Geometry: final body of the model. Coordinates: model frame, mm. A direction names the side the tool comes from. Round coordinates to 2 decimals unless told otherwise and drop trailing zeros. Write each loop counter-clockwise with the first axis right and the second up, starting at its lowest first coordinate (ties: lowest second). Pieces come first, ordered by that corner, then holes. Notation, with made-up numbers: M 23,61 L 58,61 A17 ccw 58,86 Z; hole C 62,9 d1. An arc over 180 degrees is marked long. Answer as CSV lines item,"result". Start each with the question number.
Q1. First-contact query: pin 1 (12 mm diameter, centred on x = -3.5, z = 145.5, fed in from -Y); pin 2 (6 mm diameter, centred on x = -8, z = 30.5, fed in from +Y) (3 decimals); pin 3 (1.6 mm diameter, centred on x = -1.5, y = 13.5, fed in from -Z); pin 4 (2.5 mm diameter, centred on x = -1.5, z = 53.5, fed in from +Y) (3 decimals). Flat tips, straight axial feed; report the tip coordinate or a pass-through.
Q2. Ray query, probe 1 along Y at (x, z) = (-24, 13) (3 decimals); probe 2 along X at (y, z) = (22, 149.5) (3 decimals); probe 3 along X at (y, z) = (2.1, 85). Return the intervals inside material, ascending.
Q3. Mould query, pull axis Z, two halves, no side actions, for faces 4 (the flat face through (-1.61, 23.376, 158.009)), 5 (the flat face through (-2, 14, 145)), 6 (the cylindrical face through (-13.837, 1.565, 157.615)), 7 (the flat face through (-20, 0, 84)). Classes: pulls with the +Z half, pulls with the -Z half, needs draft (parallel to the pull), parting line crosses it, or undercut.
Q4. Section query C-C on x = -9.75. Output: boundary loops of the cut face in (y, z) (3 decimals).
Q5. Reachability of faces 1 (the flat face through (-17.3, 3.175, 83.8)), 2 (the cylindrical face through (-1.565, 13.578, 154.835)), 3 (the flat face through (-2, 9, 10)) from +Z, -Z, +X, -X, +Y, -Y: full face, straight path, thin tool, end or side. Return the list, or none.
Q6. Section query D-D on z = 148. Output: boundary loops of the cut face in (x, y) (3 decimals), and give its area (3 significant figures).
Q7. Section query B-B on z = 109.5. Output: boundary loops of the cut face in (x, y) (3 decimals), and give its area (3 significant figures).
```python
from build123d import *

# Parameters (mm, degrees)
BASE_FLANGE1_DEPTH = 170
FILLET1_R          = 5
SKETCH6_R          = 2
CUT_EXTRUDE1_DEPTH = 178.200451467
SKETCH7_R          = 2.5
CUT_EXTRUDE2_DEPTH = 178.200451467
CUT_EXTRUDE3_DEPTH = 177.690635363
FILLET2_R          = 5
CUT_EXTRUDE4_DEPTH = 175.263907966
FILLET3_R          = 7


# Sheet-metal steps are written as plain solids
with BuildPart() as part:
    # Sketch1 → Base-Flange1 (new body)
    with BuildSketch(Plane.XY):
        with BuildLine():
            Line((0, 40), (0, 4.175))
            ThreePointArc((0, 4.175), (-1.222829189, 1.222829189), (-4.175, 0))
            Line((-4.175, 0), (-30, 0))
            Line((-30, 0), (-30, 3.175))
            Line((-30, 3.175), (-4.175, 3.175))
            ThreePointArc((-4.175, 3.175), (-3.467893219, 3.467893219), (-3.175, 4.175))
            Line((-3.175, 4.175), (-3.175, 40))
            Line((-3.175, 40), (0, 40))
        make_face()
    extrude(amount=BASE_FLANGE1_DEPTH)

    # Fillet1
    fillet1_edges = [part.edges().sort_by_distance(p)[0] for p in [
        (-1.5875, 40, 170),
        (-1.5875, 40, 0),
        (-30, 1.5875, 170),
        (-30, 1.5875, 0),
    ]]
    fillet(fillet1_edges, radius=FILLET1_R)

    # Sketch6 → Cut-Extrude1 (cut, through all)
    with BuildSketch(Plane.ZY):
        with BuildLine():
            ThreePointArc((159.640076561, 18.14476706), (156.999504521, 20.49580498), (154.648466601, 17.85523294))
            ThreePointArc((154.648466601, 17.85523294), (154.837103455, 13.516938304), (154.9, 9.175))
            ThreePointArc((154.9, 9.175), (157.4, 6.675), (159.9, 9.175))
            ThreePointArc((159.9, 9.175), (159.835005505, 13.661766133), (159.640076561, 18.14476706))
        make_face()
        with Locations(Location((5, 9.175, 0), (0, 0, 180))):
            Circle(SKETCH6_R)
    extrude(amount=CUT_EXTRUDE1_DEPTH, mode=Mode.SUBTRACT)

    # Sketch7 → Cut-Extrude2 (cut, through all)
    with BuildSketch(Plane.XZ):
        with Locations(Location((-14.5875, 160, 0), (0, 0, 270))):
            Circle(SKETCH7_R)
        with Locations(Location((-14.5875, 85, 0), (0, 0, 270))):
            Circle(SKETCH7_R)
        with Locations(Location((-14.5875, 10, 0), (0, 0, 270))):
            Circle(SKETCH7_R)
    extrude(amount=-CUT_EXTRUDE2_DEPTH, mode=Mode.SUBTRACT)

    # Sketch8 → Cut-Extrude3 (cut, through all)
    with BuildSketch(Plane.ZY.offset(3.175)):
        with BuildLine():
            Line((0, 12.85080004), (170, 24.175))
            Line((170, 24.175), (170, 35))
            ThreePointArc((170, 35), (168.535533906, 38.535533906), (165, 40))
            Line((165, 40), (5, 40))
            ThreePointArc((5, 40), (1.464466094, 38.535533906), (0, 35))
            Line((0, 35), (0, 12.85080004))
        make_face()
    extrude(amount=-CUT_EXTRUDE3_DEPTH, mode=Mode.SUBTRACT)

    # Fillet2
    fillet2_edges = [part.edges().sort_by_distance(p)[0] for p in [
        (-1.5875, 24.175, 170),
        (-1.5875, 12.85080004, 0),
    ]]
    fillet(fillet2_edges, radius=FILLET2_R)

    # Sketch9 → Cut-Extrude4 (cut, through all)
    with BuildSketch(Plane(origin=(0, 0, 0), x_dir=(0, 0, -1), z_dir=(1, 0, 0))):
        Polygon((-10, 13.51692945), (-145, 22.509676476), (-145, 4.175), (-10, 4.175), align=None)
    extrude(amount=-CUT_EXTRUDE4_DEPTH, mode=Mode.SUBTRACT)

    # Fillet3
    fillet3_edges = [part.edges().sort_by_distance(p)[0] for p in [
        (-1.5875, 4.175, 145),
        (-1.5875, 22.509676476, 145),
    ]]
    fillet(fillet3_edges, radius=FILLET3_R)


solid = part.part
```
Entries:
1,pin 1,"stops at y = 0"
1,pin 2,"stops at y = 3.175"
1,pin 3,"stops at z = 2.88"
1,pin 4,"stops at y = 4.175"
2,probe 1,"y = 0 to 3.175"
2,probe 2,"x = -3.175 to 0"
2,probe 3,"x = -30 to -17.09, -12.09 to -0.55"
3,face 4,"pulls with the -Z half"
3,face 5,"undercut"
3,face 6,"undercut"
3,face 7,"needs draft"
4,outline,"M 0,0 L 3.175,0 L 3.175,170 L 0,170 Z"
5,face 1,"+Z, -Z, -X, +Y"
5,face 2,"+X, -X"
5,face 3,"+X, -X, +Y"
6,outline,"M -30,0 L -4.175,0 A4.175 ccw 0,4.175 L 0,21.705 L -3.175,21.705 L -3.175,4.175 A1 cw -4.175,3.175 L -30,3.175 Z"
6,area,"151 mm^2"
7,outline,"M -30,0 L -4.175,0 A4.175 ccw 0,4.175 L -3.175,4.175 A1 cw -4.175,3.175 L -30,3.175 Z"
7,area,"94.9 mm^2"
